Geometry: final body of the model. Coordinates: model frame, mm. Give positions to 0.01 mm unless a question says otherwise; leave off trailing zeros. Write each loop counter-clockwise with the first axis right and the second up, starting at its lowest first coordinate (ties: lowest second). Pieces come first, ordered by that corner, then holes.
Q1. Section C-C (z = 3.3). Return the cut outline in (x, y).
Q2. Pin query (flat end, axial travel): pin 1 Ø1.5 at (x, z) = (-2, 3.5) entering from +Y; pin 2 Ø4.5 at (x, y) = (0, 0) entering from -Z; pin 3 Ø1 at (y, z) = (3, 3) entering from -X; pin 4 Ø1.5 at (x, z) = (-2.5, 2) entering from -Y. Return the tip coordinate at first contact, or that it passes through.
Q3. Line query: line 1 (Y direction, x = 0, z = 0.2); line 2 (Y direction, x = 1.5, z = 0.25); line 3 (Y direction, x = 0, z = 1.15). Output: solid intervals per line, ascending.
Q4. Mould query, pull axis X, two halves, no side actions, for faces 1 (the cylindrical face through (-0.54, -2.44, 1.97)), 2 (the flat face through (0, 3, 4)), 3 (the cylindrical face through (-1.08, -4.88, 1.97)). Classes: +X half, -X half, draft (parallel to the pull), parting line (faces both ways), or undercut.
from build123d import *

# Parameters (mm, degrees)
SKETCH_1_R          = 5
SKETCH_1_R_2        = 2.5
EXTRUDE_1_DEPTH     = 4
SKETCH_4_R          = 4.25
SKETCH_4_R_2        = 3.25
CUT_EXTRUDE_3_DEPTH = 0.3
SKETCH_5_R          = 4.25
SKETCH_5_R_2        = 3.25
CUT_EXTRUDE_4_DEPTH = 0.3
FILLET_2_R          = 0.2


with BuildPart() as part:
    # Эскиз1 → Бобышка-Вытянуть1 (new body)
    with BuildSketch(Plane.XY):
        Circle(SKETCH_1_R)
        Circle(SKETCH_1_R_2, mode=Mode.SUBTRACT)
    extrude(amount=EXTRUDE_1_DEPTH)

    # Эскиз4 → Вырез-Вытянуть3 (cut)
    with BuildSketch(Plane.XY.offset(4)):
        Circle(SKETCH_4_R)
        Circle(SKETCH_4_R_2, mode=Mode.SUBTRACT)
    extrude(amount=-CUT_EXTRUDE_3_DEPTH, mode=Mode.SUBTRACT)

    # Эскиз5 → Вырез-Вытянуть4 (cut)
    with BuildSketch(Plane(origin=(0, 0, 0), x_dir=(-1, 0, 0), z_dir=(0, 0, -1))):
        Circle(SKETCH_5_R)
        Circle(SKETCH_5_R_2, mode=Mode.SUBTRACT)
    extrude(amount=-CUT_EXTRUDE_4_DEPTH, mode=Mode.SUBTRACT)

    # Скругление2
    fillet_2_edges = [part.edges().sort_by_distance(p)[0] for p in [
        (-5, 0, 4),
        (-5, 0, 0),
        (-2.5, 0, 0),
        (-2.5, 0, 4),
    ]]
    fillet(fillet_2_edges, radius=FILLET_2_R)


solid = part.part
Computed:
1. outline: circle Ø10 at (0, 0); hole circle Ø5 at (0, 0)
2. pin 1: stops at y = 4.84
2. pin 2: passes through
2. pin 3: stops at x = -4.33
2. pin 4: stops at y = -4.68
3. line 1: y = -5 to -4.25, -3.25 to -2.5, 2.5 to 3.25, 4.25 to 5
3. line 2: y = -4.77 to -3.98, -2.88 to -2, 2 to 2.88, 3.98 to 4.77
3. line 3: y = -5 to -2.5, 2.5 to 5
4. face 1: undercut
4. face 2: draft
4. face 3: parting line
